from build123d import *

# Parameters (mm, degrees)
SKETCH_1_R               = 4
EXTRUDE_1_DEPTH          = 2.5
SKETCH_2_R               = 2.5
EXTRUDE_2_DEPTH          = 30
SKETCH_3_R               = 2
EXTRUDE_3_DEPTH          = 5
CUT_EXTRUDE_1_DEPTH      = 38.924266638
CUT_EXTRUDE_1_DEPTH_BACK = 1
SKETCH_4_W               = 8
SKETCH_4_H               = 1


with BuildPart() as part:
    # Sketch 1 → Extrude 1 (new body)
    with BuildSketch(Plane(origin=(0, 0, 0), x_dir=(1, 0, 0), z_dir=(0, 1, 0))):
        with Locations(Location((0, 0, 0), (0, 0, 270))):
            Circle(SKETCH_1_R)
    extrude(amount=-EXTRUDE_1_DEPTH)

    # Sketch 2 → Extrude 2 (add)
    with BuildSketch(Plane(origin=(0, 0, 0), x_dir=(1, 0, 0), z_dir=(0, 1, 0))):
        with Locations(Location((0, 0, 0), (0, 0, 270))):
            Circle(SKETCH_2_R)
    extrude(amount=EXTRUDE_2_DEPTH)

    # Sketch 3 → Extrude 3 (add)
    with BuildSketch(Plane(origin=(0, 30, 0), x_dir=(1, 0, 0), z_dir=(0, 1, 0))):
        with Locations(Location((0, 0, 0), (0, 0, 270))):
            Circle(SKETCH_3_R)
    extrude(amount=EXTRUDE_3_DEPTH)

    # Sketch 4 → Cut-Extrude 1 (cut, two sides: drawn at the far end of the back side and taken through both)
    with BuildSketch(Plane.XZ.offset(2.5).offset(-CUT_EXTRUDE_1_DEPTH_BACK)):
        Rectangle(SKETCH_4_W, SKETCH_4_H)
    extrude(amount=CUT_EXTRUDE_1_DEPTH + CUT_EXTRUDE_1_DEPTH_BACK, mode=Mode.SUBTRACT)


solid = part.part
The model under review builds one solid part; all positions refer to its coordinate system, in mm. A direction names the side the tool comes from. Round coordinates to 2 decimals unless told otherwise and drop trailing zeros. Loops run counter-clockwise (first coordinate to the right, second up) from the corner with the lowest first, then second, coordinate; pieces in that order, holes last. Notation, with made-up numbers: M 5.25,79.5 L 10.25,79.5 A23 ccw 10.25,102.5 Z; hole C 21,76 d7. An arc over 180 degrees is marked long. Answer as CSV lines item,"result". Start each with the question number.
Item 1: Consider section A-A (z = 0). Write out the cut boundary in (x, y).
Item 2: For faces 1 (the face through (0, -1.5, 0)), 2 (the face through (-2, 32, 0)), 3 (the face through (0, -2.5, -2)), list the 3-axis set-ups (+Z, -Z, +X, -X, +Y, -Y) from which the entire face can be reached by the end or side of a thin tool; tool diameter is ignored.
Item 3: Consider section D-D (x = 3.25). Write out the cut boundary in (y, z), then the cut area to 3 significant figures.
Item 4: Consider section B-B (x = 0). Write out the cut boundary in (y, z), then the cut area to 3 significant figures.
Item 5: Insertion check: P1, Ø3, axis at y = 23.5, z = 1.5, coming from the +X side; P2, Ø2, axis at y = 15, z = 2, coming from the +X side; P3, Ø0.5, axis at x = 0.5, y = -2, coming from the -Z side. Each pin has a flat end and moves straight along its axis. Give the tip position at first contact, or say it passes through.
Item 6: Consider section C-C (y = 27.5). Write out the cut boundary in (x, z).
Item 7: Wall thickness on line 1 (X direction, y = 7, z = -1.5); line 2 (Y direction, x = 1, z = 3.5): over which ranges is each line inside the solid? List them lowest first. Write a range as [from, to].
Item 8: Mouldability with a two-part tool opening along Z and no side actions: class faces 4 (the face through (0, -2, -0.5)), 5 (the face through (2, 30, -1)), 6 (the face through (0, -2, 0.5)), 7 (the face through (-2.44, 14.79, -0.54)) as released by +Z, released by -Z, zero draft, split by the parting line, or undercut.
Answer:
1,outline,"M -4,-1.5 L 4,-1.5 L 4,0 L 2.5,0 L 2.5,30 L 2,30 L 2,35 L -2,35 L -2,30 L -2.5,30 L -2.5,0 L -4,0 Z"
2,face 1,"+X, -X, -Y"
2,face 2,"+Y"
2,face 3,"+Z, -Z, +X, -X, -Y"
3,outline,"M -2.5,-2.33 L 0,-2.33 L 0,2.33 L -2.5,2.33 L -2.5,0.5 L -1.5,0.5 L -1.5,-0.5 L -2.5,-0.5 Z"
3,area,"10.7 mm^2"
4,outline,"M -2.5,-4 L 0,-4 L 0,-2.5 L 30,-2.5 L 30,-2 L 35,-2 L 35,2 L 30,2 L 30,2.5 L 0,2.5 L 0,4 L -2.5,4 L -2.5,0.5 L -1.5,0.5 L -1.5,-0.5 L -2.5,-0.5 Z"
4,area,"189 mm^2"
5,P1,"stops at x = 2.5"
5,P2,"stops at x = 2.29"
5,P3,"stops at z = -3.99"
6,outline,"C 0,0 d5"
7,line 1,"x = [-2, 2]"
7,line 2,"y = [-2.5, 0]"
8,face 4,"undercut"
8,face 5,"zero draft"
8,face 6,"undercut"
8,face 7,"split by the parting line"
